Part model, mm, in its own coordinate system. Round coordinates to 2 decimals unless told otherwise and drop trailing zeros. Write each loop counter-clockwise with the first axis right and the second up, starting at its lowest first coordinate (ties: lowest second). Pieces come first, ordered by that corner, then holes. Notation, with made-up numbers: M 33.5,69.5 L 58.5,69.5 A36 ccw 58.5,103.5 Z; hole C 21.5,7.25 d1. An arc over 180 degrees is marked long. Use a Markdown table: item, result. Add a question column.
1) Slice it at B-B on x = -14. Write the cut outline in (y, z), plus the area to 3 significant figures.
2) Drop flat-ended pins along their axis: P1, Ø1, axis at y = -1, z = -5.5, coming from the +X side; P2, Ø0.6, axis at x = -31, y = -4, coming from the +Z side. Give the stop position or say it passes through.
3) Slice it at A-A on z = -2.75. Write the cut outline in (x, y).
4) Wall check: probe 1 along X at (y, z) = (-3.9, -7.75); probe 2 along X at (y, z) = (-1.1, -2.5); probe 3 along Z at (x, y) = (-28, -5.2). Give the ranges that are in metal, low to high.
5) Slice it at C-C on y = -1.35. Write the cut outline in (x, z).
6) Slice it at D-D on z = -8.75. Write the cut outline in (x, y), plus the area to 3 significant figures.
```python
from build123d import *

# Parameters (mm, degrees)
SKETCH1_W           = 49
SKETCH1_H           = 14.8
BOSS_EXTRUDE1_DEPTH = 3.8
SKETCH2_W           = 14.6
SKETCH2_H           = 3.6
CUT_EXTRUDE1_DEPTH  = 48
SKETCH3_W           = 14.6
SKETCH3_H           = 1.5
BOSS_EXTRUDE2_DEPTH = 48
SKETCH5_W           = 2
SKETCH5_H           = 2
CUT_EXTRUDE2_DEPTH  = 2.2
FILLET1_R           = 0.5
SKETCH6_W           = 9
SKETCH6_H           = 7
BOSS_EXTRUDE3_DEPTH = 1.7
FILLET2_R           = 1


with BuildPart() as part:
    # Sketch1 → Boss-Extrude1 (new body)
    with BuildSketch(Plane(origin=(0, 0, 0), x_dir=(1, 0, 0), z_dir=(0, 1, 0))):
        with Locations((-24.5, 7.4)):
            Rectangle(SKETCH1_W, SKETCH1_H)
    extrude(amount=-BOSS_EXTRUDE1_DEPTH)

    # Sketch2 → Cut-Extrude1 (cut)
    with BuildSketch(Plane(origin=(0, 0, 0), x_dir=(0, 0, -1), z_dir=(1, 0, 0))):
        with Locations((7.4, -1.9)):
            Rectangle(SKETCH2_W, SKETCH2_H)
    extrude(amount=-CUT_EXTRUDE1_DEPTH, mode=Mode.SUBTRACT)

    # Sketch3 → Boss-Extrude2 (add)
    with BuildSketch(Plane(origin=(0, 0, 0), x_dir=(0, 0, -1), z_dir=(1, 0, 0))):
        with Locations((7.4, -2.95)):
            Rectangle(SKETCH3_W, SKETCH3_H)
    extrude(amount=-BOSS_EXTRUDE2_DEPTH)

    # Sketch5 → Cut-Extrude2 (cut)
    with BuildSketch(Plane(origin=(0, 0, 0), x_dir=(1, 0, 0), z_dir=(0, 1, 0))):
        with Locations((-6, 12.3)):
            Rectangle(SKETCH5_W, SKETCH5_H)
        with Locations((-6, 2.5)):
            Rectangle(SKETCH5_W, SKETCH5_H)
    extrude(amount=-CUT_EXTRUDE2_DEPTH, mode=Mode.SUBTRACT)

    # Fillet1
    # the kernel refuses this fillet: 0.5 mm, written as the material it takes off along each edge
    with BuildSketch(Plane(origin=(0, 1.25, 0), x_dir=(-1, 0, 0), z_dir=(0, -1, 0)), Plane(origin=(0, 1.25, -14.8), x_dir=(0, 0, 1), z_dir=(0, -1, 0))) as fillet1_piece_1:
        with BuildLine():
            CenterArc((FILLET1_R, FILLET1_R), FILLET1_R, 180, 90)
            Line((0, FILLET1_R), (0, 0))
            Line((0, 0), (FILLET1_R, 0))
        make_face()
    extrude(amount=6.3, mode=Mode.SUBTRACT)
    with BuildSketch(Plane(origin=(-49, 1.25, -14.8), x_dir=(0, 0, 1), z_dir=(0, -1, 0)), Plane(origin=(-49, 1.25, 0), x_dir=(1, 0, 0), z_dir=(0, -1, 0))) as fillet1_piece_2:
        with BuildLine():
            CenterArc((FILLET1_R, -FILLET1_R), FILLET1_R, 90, 90)
            Line((0, -FILLET1_R), (0, 0))
            Line((0, 0), (FILLET1_R, 0))
        make_face()
    extrude(amount=6.3, mode=Mode.SUBTRACT)

    # Sketch6 → Boss-Extrude3 (add)
    with BuildSketch(Plane.XZ.offset(3.8)):
        with Locations((-29.5, -7.4)):
            Rectangle(SKETCH6_W, SKETCH6_H)
    extrude(amount=BOSS_EXTRUDE3_DEPTH)

    # Fillet2
    fillet2_edges = [part.edges().sort_by_distance(p)[0] for p in [
        (-34, -5.5, -7.4),
        (-29.5, -5.5, -10.9),
        (-25, -5.5, -7.4),
        (-29.5, -5.5, -3.9),
    ]]
    fillet(fillet2_edges, radius=FILLET2_R)


solid = part.part
```
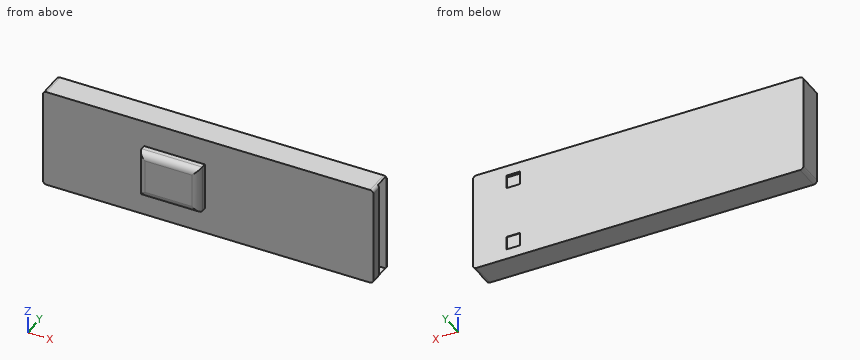
Entries:
| question | item | result |
|---|---|---|
| 1 | outline | M -3.8,-14.8 L 0,-14.8 L 0,0 L -3.8,0 Z; hole M -2.2,-14.7 L -0.1,-14.7 L -0.1,-0.1 L -2.2,-0.1 Z |
| 1 | area | 25.6 mm^2 |
| 2 | P1 | stops at x = -48 |
| 2 | P2 | stops at z = 0 |
| 3 | outline | M -49,-3.8 L 0,-3.8 L 0,-2.2 L -48,-2.2 L -48,-0.1 L -7,-0.1 L -7,0 L -49,0 Z; M -5,-0.1 L 0,-0.1 L 0,0 L -5,0 Z |
| 4 | probe 1 | x = -34 to -25 |
| 4 | probe 2 | x = -49 to -48 |
| 4 | probe 3 | z = -10.61 to -4.19 |
| 5 | outline | M -49,-14.3 A0.5 ccw -48.5,-14.8 L -0.5,-14.8 A0.5 ccw -0.2,-14.7 L -48,-14.7 L -48,-0.1 L -0.2,-0.1 A0.5 ccw -0.5,0 L -48.5,0 A0.5 ccw -49,-0.5 Z |
| 6 | outline | M -49,-3.8 L -34,-3.8 L -34,-4.5 A1 ccw -33,-5.5 L -26,-5.5 A1 ccw -25,-4.5 L -25,-3.8 L 0,-3.8 L 0,-2.2 L -48,-2.2 L -48,-0.1 L 0,-0.1 L 0,0 L -49,0 Z |
| 6 | area | 100 mm^2 |
